Job drawing, mm, ordinate dimensions from the low corner. One solid piece. Give positions to 0.01 mm unless a question says otherwise; leave off trailing zeros. Loops run counter-clockwise (first coordinate to the right, second up) from the corner with the lowest first, then second, coordinate; pieces in that order, holes last. Notation, with made-up numbers: M 46.5,-23.75 L 67.5,-23.75 A28 ccw 67.5,-0.75 Z; hole C -6,-35 d5. An arc over 180 degrees is marked long. Put each result on its own line as item: value.
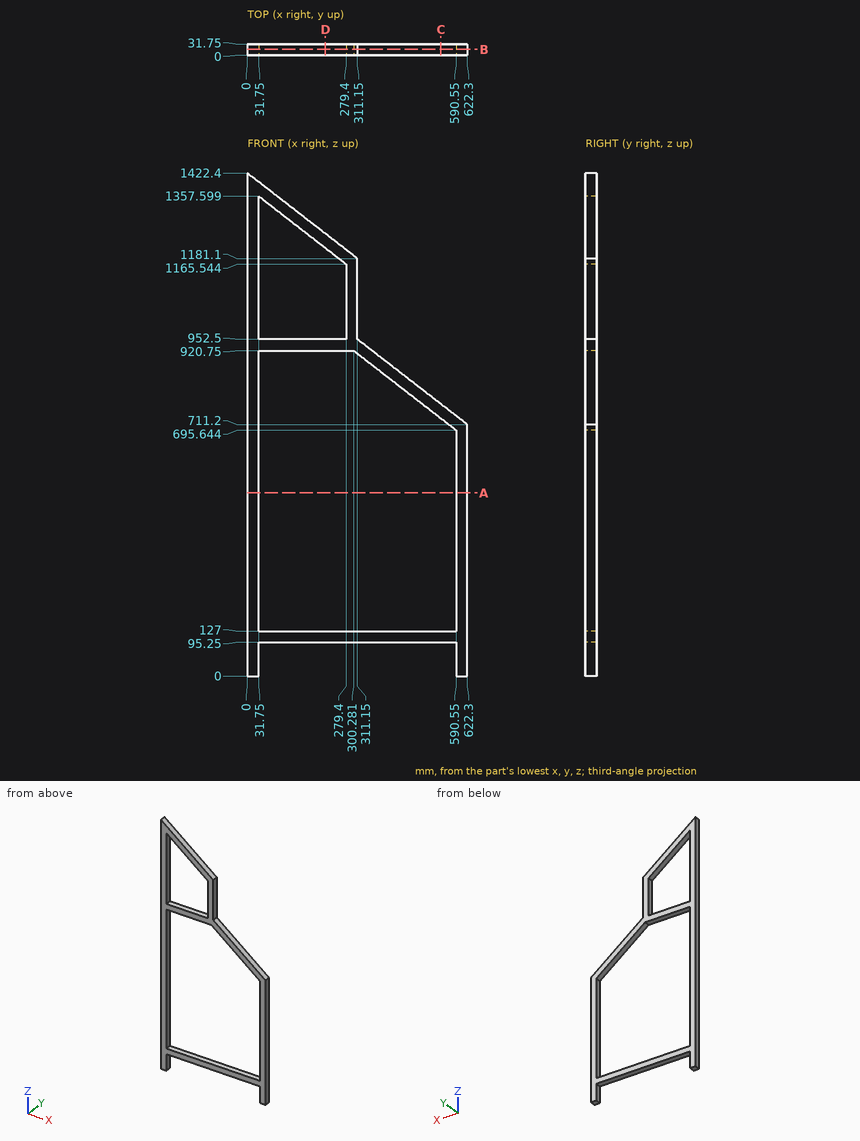
Q1. Slice it at B-B (y = 16.5). List the corners of the cut face in (x, z), and give its area (3 significant figures).
Here are the results:
outline: M 0,0 L 31.75,0 L 31.75,95.25 L 590.55,95.25 L 590.55,0 L 622.3,0 L 622.3,711.2 L 311.15,952.5 L 311.15,1181.1 L 0,1422.4 Z; hole M 31.75,127 L 590.55,127 L 590.55,695.64 L 300.28,920.75 L 31.75,920.75 Z; hole M 31.75,952.5 L 279.4,952.5 L 279.4,1165.54 L 31.75,1357.6 Z
area: 123,000 mm²
Q2. Slice it at C-C (x = 547). List the corners of the cut face in (y, z), and give its area (3 significant figures).
Here are the results:
outline: M 0,95.25 L 31.75,95.25 L 31.75,127 L 0,127 Z; M 0,729.42 L 31.75,729.42 L 31.75,769.6 L 0,769.6 Z
area: 2,280 mm²
Q3. Slice it at A-A (z = 518). List the corners of the cut face in (x, y), and give its area (3 significant figures).
Here are the results:
outline: M 0,0 L 31.75,0 L 31.75,31.75 L 0,31.75 Z; M 590.55,0 L 622.3,0 L 622.3,31.75 L 590.55,31.75 Z
area: 2,020 mm²
Q4. Drop flat-ended pins along their axis: pin 1 Ø16 at (x, y) = (133.5, 15) entering from +Z; pin 2 Ø1.5 at (x, y) = (276.5, 23.5) entering from +Z; pin 3 Ø16 at (x, y) = (213.5, 8) entering from +Z. Give the stop position or say it passes through.
Here are the results:
pin 1: z = 1325.07
pin 2: z = 1208.55
pin 3: z = 1263.03
Q5. Probe line 1 (X direction, y = 20, z = 538); line 2 (Z direction, x = 269.5, y = 26.5); line 3 (X direction, y = 13, z = 1052). List the from-to ranges inside material, lowest first. Write a range as from..to.
Here are the results:
line 1: 0..31.75, 590.55..622.3
line 2: 95.25..127, 920.75..952.5, 1173.22..1213.4
line 3: 0..31.75, 279.4..311.15
Q6. Slice it at D-D (x = 220.5). List the corners of the cut face in (y, z), and give its area (3 significant figures).
Here are the results:
outline: M 0,95.25 L 31.75,95.25 L 31.75,127 L 0,127 Z; M 0,920.75 L 31.75,920.75 L 31.75,952.5 L 0,952.5 Z; M 0,1211.22 L 31.75,1211.22 L 31.75,1251.4 L 0,1251.4 Z
area: 3,290 mm²
